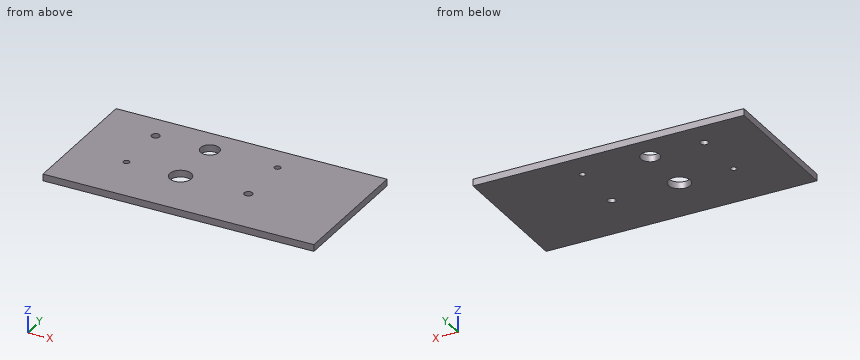
```python
from build123d import *

# Parameters (mm, degrees)
F0_W     = 127
F0_H     = 63.5
F1_DEPTH = 3.175
F3_D     = 3.7973
F4_D     = 2.8702
F5_D     = 8.73125
F6_D     = 10.0838


# Not quite as in the source:
# - a length typed as a fraction of an inch, garbled in the dataset ("3 / 203.2 mm" for 3/8 in), is restored


with BuildPart() as f1:
    # F0 (on Top) → F1 (new body)
    with BuildSketch(Plane.XY):
        with Locations((63.5, 31.75)):
            Rectangle(F0_W, F0_H)
    extrude(amount=F1_DEPTH)

    # F3 (through all)
    with Locations(Plane.XY.offset(3.175)):
        with Locations((25.4, 50.8), (82.55, 25.4)):
            Hole(F3_D / 2)

    # F4 (through all)
    with Locations(Plane.XY.offset(3.175)):
        with Locations((25.4, 25.4), (82.55, 50.8)):
            Hole(F4_D / 2)

    # F5 (through all)
    with Locations(Plane.XY.offset(3.175)):
        with Locations((50.8, 50.8)):
            Hole(F5_D / 2)

    # F6 (through all)
    with Locations(Plane.XY.offset(3.175)):
        with Locations((50.8, 25.4)):
            Hole(F6_D / 2)


solid = f1.part
```
The listing builds one solid part. Answer for the finished solid, in the listing's coordinates (mm). Coordinates: 2 decimals unless noted, no trailing zeros. Write each loop counter-clockwise with the first axis right and the second up, starting at its lowest first coordinate (ties: lowest second). Pieces come first, ordered by that corner, then holes. Notation, with made-up numbers: (22, -40) - (41, -40) arc R4 ccw to (41, -34) - close; hole circle Ø8 at (18.5, 58.5). An arc over 180 degrees is marked (long way). Return JSON: item names as keys, results as strings. Group by question number.
1. A cutting plane is placed at B-B, the plane x = 82.55. Determine the outline of the cut face in (y, z) (3 decimals).
2. A cutting plane is placed at A-A, the plane y = 25.4. Determine the outline of the cut face in (x, z) (3 decimals), plus the area to 3 significant figures.
3. Straight lines are drawn through the part: L1, parallel to X at y = 25.5, z = 1.9; L2, parallel to Y at x = 82.55, z = 2.1; L3, parallel to Y at x = 50.8, z = 1.7. For each, find the intervals that lie inside material, in ascending order.
4. Given pin 1 (3.5 mm diameter, centred on x = 25.4, y = 25.4, fed in from +Z) (3 decimals), flat-ended and moving along its own axis, determine where the tip first touches the part or whether it passes through.
5. A cutting plane is placed at C-C, the plane z = 2.1. Determine the outline of the cut face in (x, y).
6. A cutting plane is placed at D-D, the plane x = 50.8. Determine the outline of the cut face in (y, z) (3 decimals), plus the area to 3 significant figures.
Ans:
{
 "1": {"outline": "(0, 0) - (23.501, 0) - (23.501, 3.175) - (0, 3.175) - close; (27.299, 0) - (49.365, 0) - (49.365, 3.175) - (27.299, 3.175) - close; (52.235, 0) - (63.5, 0) - (63.5, 3.175) - (52.235, 3.175) - close"},
 "2": {"outline": "(0, 0) - (23.965, 0) - (23.965, 3.175) - (0, 3.175) - close; (26.835, 0) - (45.758, 0) - (45.758, 3.175) - (26.835, 3.175) - close; (55.842, 0) - (80.651, 0) - (80.651, 3.175) - (55.842, 3.175) - close; (84.449, 0) - (127, 0) - (127, 3.175) - (84.449, 3.175) - close", "area": "350 mm²"},
 "3": {"L1": "0 to 23.97, 26.83 to 45.76, 55.84 to 80.65, 84.45 to 127", "L2": "0 to 23.5, 27.3 to 49.36, 52.24 to 63.5", "L3": "0 to 20.36, 30.44 to 46.43, 55.17 to 63.5"},
 "4": {"pin 1": "z = 3.175"},
 "5": {"outline": "(0, 0) - (127, 0) - (127, 63.5) - (0, 63.5) - close; hole circle Ø3.8 at (25.4, 50.8); hole circle Ø2.87 at (25.4, 25.4); hole circle Ø10.08 at (50.8, 25.4); hole circle Ø8.73 at (50.8, 50.8); hole circle Ø3.8 at (82.55, 25.4); hole circle Ø2.87 at (82.55, 50.8)"},
 "6": {"outline": "(0, 0) - (20.358, 0) - (20.358, 3.175) - (0, 3.175) - close; (30.442, 0) - (46.434, 0) - (46.434, 3.175) - (30.442, 3.175) - close; (55.166, 0) - (63.5, 0) - (63.5, 3.175) - (55.166, 3.175) - close", "area": "142 mm²"}
}
